The model under review builds one solid part; all positions refer to its coordinate system, in mm. Face numbers are marked on the shaded views. A direction names the side the tool comes from. Give positions to 0.01 mm unless a question says otherwise; leave off trailing zeros. Order: outer loops, then holes, each group sorted by start corner. A loop starts at its lowest first (then second) coordinate and runs counter-clockwise, first axis right, second up. Notation, with made-up numbers: M -21.75,31 L -3.75,31 A15 cw -3.75,48 Z; hole C 73.5,73 d9. An arc over 180 degrees is marked long. One line per question, with ' | ' between items. Start each with the question number.
1. For the marked faces 4, 5 and 6, list the 3-axis set-ups (+Z, -Z, +X, -X, +Y, -Y) from which the entire face can be reached by the end or side of a thin tool; tool diameter is ignored.
2. We need section C-C on x = 32.5. Write out the cut boundary in (y, z).
3. The part is to be moulded in two halves that separate along Z. For the marked faces 1, 2 and 3, say which applies: +Z half, -Z half, draft (parallel to the pull), parting line (faces both ways), or undercut.
4. Insertion check: P1, Ø1.5, axis at x = 79, z = -16, coming from the -Y side; P2, Ø1.5, axis at x = 34.5, z = 10.5, coming from the +Y side; P3, Ø1, axis at x = 15, z = 6, coming from the -Y side. Each pin has a flat end and moves straight along its axis. Give the tip position at first contact, or say it passes through.
5. Wall thickness on L1, parallel to Z at x = 62, y = 0; L2, parallel to Y at x = 119.5, z = -0.5: over which ranges is each line inside the solid? List them lowest first.
6. We need section D-D on x = 112. Write out the cut boundary in (y, z), then the cut area to 3 significant figures.
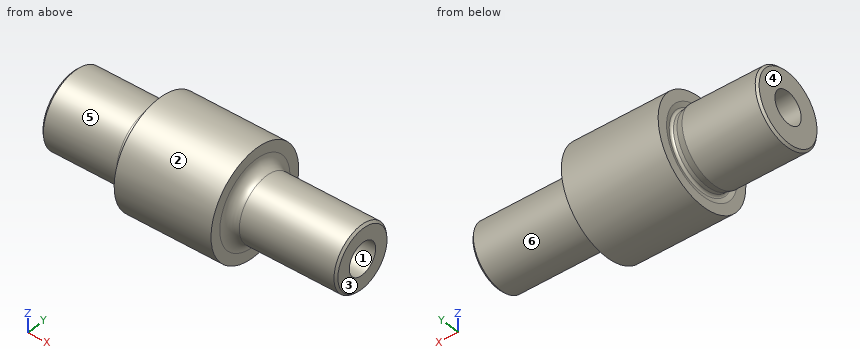
```python
from build123d import *

# Parameters (mm, degrees)
F2_SIZE = 1
F3_R    = 5


with BuildPart() as f1:
    # F0 (on Front) → F1 (revolve)
    with BuildSketch(Plane.XZ):
        with BuildLine():
            Line((0, 17.5), (0, 7.5))
            Line((0, 7.5), (135, 7.5))
            Line((135, 7.5), (135, 15))
            Line((135, 15), (85, 15))
            Line((85, 15), (85, 25))
            Line((85, 25), (40, 25))
            Line((40, 25), (40, 20.2))
            Line((40, 20.2), (40.600523, 17.958819))
            ThreePointArc((40.600523, 17.958819), (40.42795, 17.091239), (39.634597, 16.7))
            Line((39.634597, 16.7), (37.985641, 16.7))
            Line((37.985641, 16.7), (35, 17.5))
            Line((35, 17.5), (0, 17.5))
        make_face()
    revolve(axis=Axis((67.5, 0, 0), (1, 0, 0)))

    # F2
    f2_edges = [f1.edges().sort_by_distance(p)[0] for p in [
        (0, 0, -17.5),
        (135, 0, -15),
    ]]
    chamfer(f2_edges, length=F2_SIZE)

    # F3
    f3_edges = [f1.edges().sort_by_distance(p)[0] for p in [
        (85, 0, -15),
    ]]
    fillet(f3_edges, radius=F3_R)


solid = f1.part
```
Entries:
1) face 4: +Z, -Z, -X, +Y, -Y | face 5: -X | face 6: +X
2) outline: C 0,0 d35; hole C 0,0 d15
3) face 1: undercut | face 2: parting line | face 3: draft
4) P1: stops at y = -19.81 | P2: stops at y = 14.53 | P3: stops at y = -16.61
5) L1: z = -25 to -7.5, 7.5 to 25 | L2: y = -14.99 to -7.48, 7.48 to 14.99
6) outline: C 0,0 d30; hole C 0,0 d15 | area: 530 mm^2
